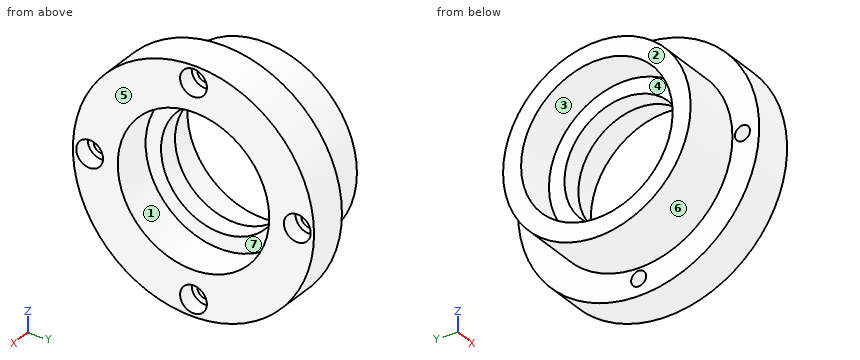
```python
from build123d import *

# Parameters (mm, degrees)
CBORE_FOR_M4_SHCS1_D           = 4.5
CBORE_FOR_M4_SHCS1_CBORE_D     = 8
CBORE_FOR_M4_SHCS1_CBORE_DEPTH = 5
CIRPATTERN1_COUNT              = 4


with BuildPart() as part:
    # Sketch1 → Revolve1 (revolve)
    with BuildSketch(Plane.XY):
        Polygon((-30, 22.621875), (-18, 22.621875), (-18, 18), (-12, 18), (-12, 22.621875), (0, 22.621875), (0, 36), (-12, 36), (-12, 28), (-30, 28), align=None)
    revolve(axis=Axis((-59.7296875, 0, 0), (1, 0, 0)))

    # CBORE for M4 SHCS1 (through all)
    with Locations(Plane(origin=(0, 0, 0), x_dir=(0, 0, -1), z_dir=(1, 0, 0))):
        with Locations((0, 31)):
            cbore_for_m4_shcs1 = CounterBoreHole(CBORE_FOR_M4_SHCS1_D / 2, CBORE_FOR_M4_SHCS1_CBORE_D / 2, CBORE_FOR_M4_SHCS1_CBORE_DEPTH)

    # CirPattern1: CBORE for M4 SHCS1 ×4 about axis
    cirpattern1_axis = Axis((0, 0, 0), (1, 0, 0))
    for i in range(1, CIRPATTERN1_COUNT):
        add(cbore_for_m4_shcs1.rotate(cirpattern1_axis, i * 360 / CIRPATTERN1_COUNT), mode=Mode.SUBTRACT)


solid = part.part
```
Check sheet for the modelled part. Datum: model origin and axes. Units: mm. Face numbers are marked on the shaded views. A direction names the side the tool comes from. Give positions to 0.01 mm unless a question says otherwise; leave off trailing zeros. Write each loop counter-clockwise with the first axis right and the second up, starting at its lowest first coordinate (ties: lowest second). Pieces come first, ordered by that corner, then holes. Notation, with made-up numbers: (83.5, -31) -> (94.5, -31) arc R10 cw to (94.5, -23) -> close; hole circle Ø1 at (62.5, -3.5). An arc over 180 degrees is marked (long way). Use CSV: the item, a comma, the result in double quotes. Start each with the question number.
Q1. Depth check by flat-ended pin: P1, Ø5, axis at y = 0, z = -31, coming from the +X side; P2, Ø5, axis at y = 0, z = 31, coming from the -X side; P3, Ø1, axis at x = -12, z = -4.5, coming from the +Y side; P4, Ø9, axis at y = -1.5, z = 30.5, coming from the +X side. Enter the tip coordinate at first touch or a pass-through.
Q2. Tool access check on the marked faces 1, 2 and 3. Record the directions out of +Z, -Z, +X, -X, +Y, -Y that give a thin tool (end or side, any length) a straight path to the whole face; none if there is none.
Q3. Cross-section at B-B on x = -7.5. Enter the section's corners in (y, z), and give its area (3 significant figures).
Q4. Release check for a two-part mould opening along Y. For the marked faces 4, 5, 6 and 7 record: +Y half, -Y half, draft (parallel to the pull), parting line (faces both ways), or undercut.
Q5. Scan lines: line 1 along Z through (x, y) = (-2.85, 0); line 2 along Z through (x, y) = (-7, 0); line 3 along Z through (x, y) = (-16.6, 0). Record each from-to range of solid material in increasing order.
Q6. Cross-section at D-D on x = -22.5. Enter the section's corners in (y, z), and give its area (3 significant figures).
Q7. Cross-section at A-A on y = -31. Enter the section's corners in (x, z).
Working result:
1,P1,"stops at x = -5"
1,P2,"stops at x = -12"
1,P3,"stops at y = 35.78"
1,P4,"stops at x = 0"
2,face 1,"+X"
2,face 2,"+Z, -Z, -X, +Y, -Y"
2,face 3,"-X"
3,outline,"circle Ø72 at (0, 0); hole circle Ø4.5 at (-31, 0); hole circle Ø45.24 at (0, 0); hole circle Ø4.5 at (0, -31); hole circle Ø4.5 at (0, 31); hole circle Ø4.5 at (31, 0)"
3,area,"2,400 mm^2"
4,face 4,"undercut"
4,face 5,"draft"
4,face 6,"parting line"
4,face 7,"undercut"
5,line 1,"z = -36 to -35, -27 to -22.62, 22.62 to 27, 35 to 36"
5,line 2,"z = -36 to -33.25, -28.75 to -22.62, 22.62 to 28.75, 33.25 to 36"
5,line 3,"z = -28 to -18, 18 to 28"
6,outline,"circle Ø56 at (0, 0); hole circle Ø45.24 at (0, 0)"
6,area,"855 mm^2"
7,outline,"(-12, -18.3) -> (0, -18.3) -> (0, -4) -> (-5, -4) -> (-5, -2.25) -> (-12, -2.25) -> close; (-12, 2.25) -> (-5, 2.25) -> (-5, 4) -> (0, 4) -> (0, 18.3) -> (-12, 18.3) -> close"
